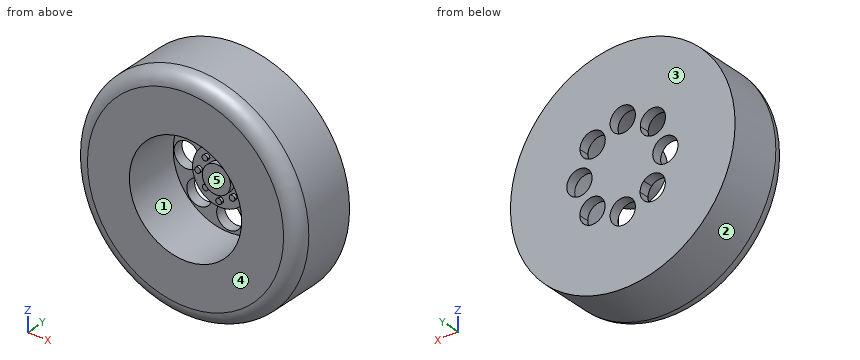
```python
from build123d import *

# Parameters (mm, degrees)
F0_R      = 20
F1_DEPTH  = 12
F2_R      = 2.54
F3_R      = 10
F4_DEPTH  = 10.16
F5_R      = 5
F6_DEPTH  = 2
F7_R      = 2.5
F8_DEPTH  = 1
F10_R     = 2.25
F12_DEPTH = 25.4
F13_DEPTH = 25.4
F14_R     = 0.5
F15_DEPTH = 0.5


with BuildPart() as f1:
    # F0 (on Front) → F1 (new body)
    with BuildSketch(Plane.XZ):
        Circle(F0_R)
    extrude(amount=F1_DEPTH)

    # F2
    f2_edges = [f1.edges().sort_by_distance(p)[0] for p in [
        (-20, -12, 0),
    ]]
    fillet(f2_edges, radius=F2_R)

    # F3 (on face) → F4 (cut)
    with BuildSketch(Plane.XZ.offset(12)):
        Circle(F3_R)
    extrude(amount=-F4_DEPTH, mode=Mode.SUBTRACT)

    # F5 (on face) → F6 (join)
    with BuildSketch(Plane.XZ.offset(1.84)):
        Circle(F5_R)
    extrude(amount=F6_DEPTH)

    # F7 (on face) → F8 (join)
    with BuildSketch(Plane.XZ.offset(3.84)):
        Circle(F7_R)
    extrude(amount=F8_DEPTH)

    # F10 (on face) → F12 (cut)
    with BuildSketch(Plane.XZ.offset(1.84)):
        with Locations((0, 7.612496)):
            Circle(F10_R)
        with Locations((7.716608, 0)):
            Circle(F10_R)
        with Locations((0, -7.387504)):
            Circle(F10_R)
        with Locations((-7.583391, 0)):
            Circle(F10_R)
    extrude(amount=-F12_DEPTH, mode=Mode.SUBTRACT)

    # F11 (on face) → F13 (cut)
    with BuildSketch(Plane.XZ.offset(1.84)):
        with BuildLine():
            ThreePointArc((7.612273, 5.362273), (4.501235, 7.441002), (3.771282, 3.771282))
            ThreePointArc((3.771282, 3.771282), (6.22331, 3.283544), (7.612273, 5.362273))
        make_face()
        with BuildLine():
            ThreePointArc((-3.112273, 5.362273), (-7.441002, 6.22331), (-3.771282, 3.771282))
            ThreePointArc((-3.771282, 3.771282), (-3.283544, 4.501235), (-3.112273, 5.362273))
        make_face()
        with BuildLine():
            ThreePointArc((-3.078865, -5.328865), (-3.250136, -4.467827), (-3.737875, -3.737875))
            ThreePointArc((-3.737875, -3.737875), (-7.407594, -6.189903), (-3.078865, -5.328865))
        make_face()
        with BuildLine():
            ThreePointArc((7.645473, -5.395473), (6.256511, -3.316744), (3.804483, -3.804483))
            ThreePointArc((3.804483, -3.804483), (4.534436, -7.474202), (7.645473, -5.395473))
        make_face()
    extrude(amount=-F13_DEPTH, mode=Mode.SUBTRACT)

    # F14 (on face) → F15 (join)
    with BuildSketch(Plane.XZ.offset(3.84)):
        with BuildLine():
            ThreePointArc((0.5, 3.70109), (-0.353553, 4.054643), (0, 3.20109))
            ThreePointArc((0, 3.20109), (0.353553, 3.347536), (0.5, 3.70109))
        make_face()
        with BuildLine():
            ThreePointArc((3.017969, 2.517969), (2.326627, 2.979909), (2.164415, 2.164415))
            ThreePointArc((2.164415, 2.164415), (2.709311, 2.056029), (3.017969, 2.517969))
        make_face()
        with BuildLine():
            ThreePointArc((4.305301, 0), (3.805301, 0.5), (3.305301, 0))
            ThreePointArc((3.305301, 0), (3.805301, -0.5), (4.305301, 0))
        make_face()
        with BuildLine():
            ThreePointArc((2.904961, -2.404961), (2.596303, -1.943022), (2.051408, -2.051408))
            ThreePointArc((2.051408, -2.051408), (2.21362, -2.866901), (2.904961, -2.404961))
        make_face()
        with BuildLine():
            ThreePointArc((0.5, -3.792667), (0.353553, -3.439113), (0, -3.292667))
            ThreePointArc((0, -3.292667), (-0.353553, -4.14622), (0.5, -3.792667))
        make_face()
        with BuildLine():
            ThreePointArc((-1.850414, -2.350414), (-1.888474, -2.159072), (-1.99686, -1.99686))
            ThreePointArc((-1.99686, -1.99686), (-2.812353, -2.541755), (-1.850414, -2.350414))
        make_face()
        with Locations((-3.738696, 0)):
            Circle(F14_R)
        with BuildLine():
            ThreePointArc((-1.941345, 2.441345), (-2.903285, 2.632687), (-2.087792, 2.087792))
            ThreePointArc((-2.087792, 2.087792), (-1.979406, 2.250004), (-1.941345, 2.441345))
        make_face()
    extrude(amount=F15_DEPTH)


solid = f1.part
```
Could you check a few things on this model? Use its own coordinates, in mm. Face numbers are marked on the shaded views. A direction names the side the tool comes from. Coordinates: 2 decimals unless noted, no trailing zeros. Loops run counter-clockwise (first coordinate to the right, second up) from the corner with the lowest first, then second, coordinate; pieces in that order, holes last. Notation, with made-up numbers: M -34.5,41 L 18.5,41 A23 cw 18.5,51 Z; hole C 60,36 d7. An arc over 180 degrees is marked long. Put each result on its own line as item: value. Start each with the question number.
(1) I need wall thicknesses on line 1 (Z direction, x = 0, y = -1.4); line 2 (Z direction, x = 0, y = -5.75); line 3 (Z direction, x = -4, y = -0.75). Which ranges of each line are inside material? Lowest first, please. Write a range as from..to.
(2) Thinking about a two-plate mould opening in X: for the marked faces 1, 2 and 3, which applies, pulls with the +X half, pulls with the -X half, needs draft (parallel to the pull), parting line crosses it, or undercut?
(3) Suppose I cut it at A-A on z = 0. Count the separate pieces of the cut face and the enclosed holes in it, then the cut area to 3 significant figures.
(4) For the marked faces 4 and 5, which set-ups out of +Z, -Z, +X, -X, +Y, -Y let a thin tool reach every point of the face, with its end or its side?
(5) Suppose I cut it at D-D on y = -10. Please give me the cut outline in (x, z), then the cut area to 3 significant figures.
(6) Will these pins go through, and if not, where does the flat tip stop? P1, Ø5, axis at x = 0, z = 7.61, coming from the +Y side; P2, Ø5, axis at x = -0.5, z = 0.5, coming from the -Y side; P3, Ø1, axis at x = -14.5, y = -7, coming from the -Z side; P4, Ø3, axis at x = 2.5, y = -4.5, coming from the +Z side (3 decimals).
Solutions:
1. line 1: z = -20..-9.64, -5.14..5.36, 9.86..20
1. line 2: z = -20..-10, 10..20
1. line 3: z = -19.6..-7.14, -3.51..3.57, 7.15..19.6
2. face 1: undercut
2. face 2: parting line crosses it
2. face 3: needs draft
3. separate pieces: 3
3. enclosed holes: 0
3. area: 283 mm2
4. face 4: +Z, -Z, +X, -X, -Y
4. face 5: -Y
5. outline: C 0,0 d39.88; hole C 0,0 d20
5. area: 935 mm2
6. P1: stops at y = 0
6. P2: stops at y = -4.84
6. P3: stops at z = -14.28
6. P4: stops at z = 19.975
